For this review, use the dimensioned drawing (mm, ordinates from the lowest corner) and the shaded views. A direction names the side the tool comes from. Coordinates: 2 decimals unless noted, no trailing zeros. Loops run counter-clockwise (first coordinate to the right, second up) from the corner with the lowest first, then second, coordinate; pieces in that order, holes last.
1. To check wall thickness, follow probe 1 along X at (y, z) = (6.5, 7.5); probe 2 along Y at (x, z) = (59.75, 17.5) (3 decimals); probe 3 along Y at (x, z) = (30, 14). State the ranges of each line that lie inside material, in increasing order.
2. Clearance check with flat-ended pins moving along their axes: P1, Ø1, axis at y = 19.5, z = 22, coming from the -X side; P2, Ø6, axis at x = 43.5, z = 14.5, coming from the +Y side. State where each tip first meets the part, or that it passes through.
3. Take a section at B-B, the plane y = 10.5. State the section outline as (x, z) points.
4. Mouldability with a two-part tool opening along X and no side actions: class the marked faces 1, 2, 3 and 4 as pulls with the +X half, pulls with the -X half, needs draft (parallel to the pull), parting line crosses it, or undercut.
5. Take a section at A-A, the plane z = 17.5. State the section outline as (x, y) points (3 decimals), then the cut area to 3 significant figures.
6. Take a section at C-C, the plane z = 23.5. State the section outline as (x, y) points (3 decimals).
7. Take a section at D-D, the plane x = 50.5. State the section outline as (y, z) points, then the cut area to 3 significant figures.
8. Machinability: for the marked faces 5 and 6, which of the approach directions +Z, -Z, +X, -X, +Y, -Y give a long, thin tool a straight path to every point of the face, cutting with its end or side? Answer none if there is none.
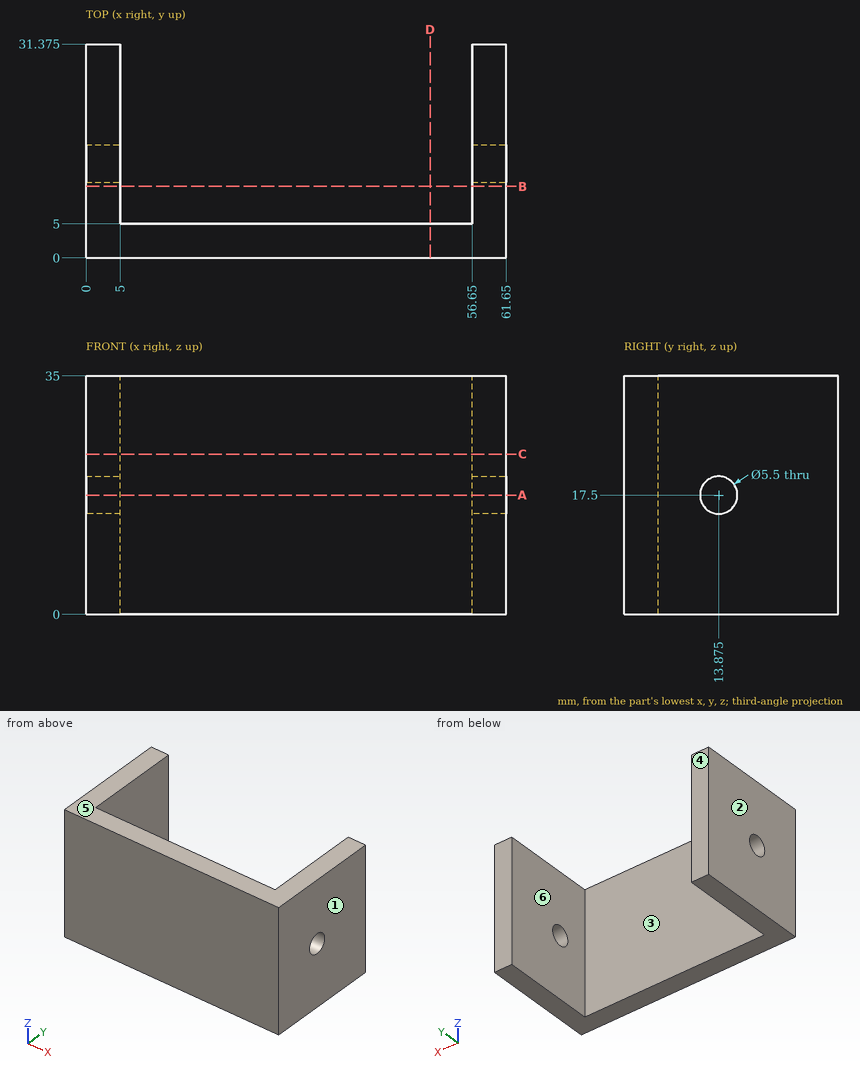
Results list:
1. probe 1: x = 0 to 5, 56.65 to 61.65
1. probe 2: y = 0 to 11.125, 16.625 to 31.375
1. probe 3: y = 0 to 5
2. P1: stops at x = 0
2. P2: stops at y = 5
3. outline: (0, 0) - (5, 0) - (5, 35) - (0, 35) - close; (56.65, 0) - (61.65, 0) - (61.65, 35) - (56.65, 35) - close
4. face 1: pulls with the +X half
4. face 2: pulls with the -X half
4. face 3: undercut
4. face 4: needs draft
5. outline: (0, 0) - (61.65, 0) - (61.65, 11.125) - (56.65, 11.125) - (56.65, 5) - (5, 5) - (5, 11.125) - (0, 11.125) - close; (0, 16.625) - (5, 16.625) - (5, 31.375) - (0, 31.375) - close; (56.65, 16.625) - (61.65, 16.625) - (61.65, 31.375) - (56.65, 31.375) - close
5. area: 517 mm2
6. outline: (0, 0) - (61.65, 0) - (61.65, 31.375) - (56.65, 31.375) - (56.65, 5) - (5, 5) - (5, 31.375) - (0, 31.375) - close
7. outline: (0, 0) - (5, 0) - (5, 35) - (0, 35) - close
7. area: 175 mm2
8. face 5: +Z, +X, -X, +Y, -Y
8. face 6: +Z, -Z, +Y
